from build123d import *

# Parameters (mm, degrees)
BOSS_EXTRUDE1_DEPTH     = 50.8
BOSS_EXTRUDE1_2_DEPTH   = 50.8
BOSS_EXTRUDE2_START     = 50.8
BOSS_EXTRUDE2_DEPTH     = 5.08
F_1_4_CLEARANCE_HOLE1_D = 6.7564
F_1_4_CLEARANCE_HOLE2_D = 6.7564


with BuildPart() as part:
    # Sketch1 → Boss-Extrude1 (new body, symmetric)
    with BuildSketch(Plane.XY):
        with BuildLine():
            ThreePointArc((-13.252570374, 55.853277384), (-42.992049277, 38.038177072), (-57.051702131, 6.35))
            Line((-57.051702131, 6.35), (-70.104, 6.35))
            Line((-70.104, 6.35), (-70.104, 0))
            Line((-70.104, 0), (-51.203999954, 0))
            ThreePointArc((-51.203999954, 0), (-40.6228644, 31.171020183), (-13.252570374, 49.459265965))
            Line((-13.252570374, 49.459265965), (-13.252570374, 55.853277384))
        make_face()
    extrude(amount=BOSS_EXTRUDE1_DEPTH, both=True)



with BuildPart() as body_2:
    # Sketch1 → Boss-Extrude1 2 (new body, symmetric)
    with BuildSketch(Plane.XY):
        with BuildLine():
            Line((13.252570374, 55.853277384), (13.252570374, 49.459265965))
            ThreePointArc((13.252570374, 49.459265965), (37.75154872, 34.59292096), (50.42609614, 8.891481281))
            Line((50.42609614, 8.891481281), (70.104, 8.891481281))
            Line((70.104, 8.891481281), (70.104, 15.241481281))
            Line((70.104, 15.241481281), (55.343621713, 15.241481281))
            ThreePointArc((55.343621713, 15.241481281), (39.858360326, 41.310172211), (13.252570374, 55.853277384))
        make_face()
    extrude(amount=BOSS_EXTRUDE1_2_DEPTH, both=True)


with BuildPart() as part_1:
    add(part.part)

    add(body_2.part)  # Boss-Extrude2 merges body 2
    # Sketch1<4> → Boss-Extrude2 (add)
    with BuildSketch(Plane.XY.offset(BOSS_EXTRUDE2_START)):
        with BuildLine():
            Line((-13.252570374, 55.853277384), (-13.252570374, 49.459265965))
            ThreePointArc((-13.252570374, 49.459265965), (0, 51.203999954), (13.252570374, 49.459265965))
            Line((13.252570374, 49.459265965), (13.252570374, 55.853277384))
            ThreePointArc((13.252570374, 55.853277384), (0, 57.404), (-13.252570374, 55.853277384))
        make_face()
    extrude(amount=-BOSS_EXTRUDE2_DEPTH)

    # 1/4 Clearance Hole1 (through all)
    with Locations(Plane(origin=(0, 6.35, 0), x_dir=(1, 0, 0), z_dir=(0, 1, 0))):
        with Locations((-62.484, -31.75), (-62.484, 31.75)):
            Hole(F_1_4_CLEARANCE_HOLE1_D / 2)

    # 1/4 Clearance Hole2 (through all)
    with Locations(Plane(origin=(0, 15.241481281, 0), x_dir=(1, 0, 0), z_dir=(0, 1, 0))):
        with Locations((62.484, -31.75), (62.484, 31.75)):
            Hole(F_1_4_CLEARANCE_HOLE2_D / 2)


solid = part_1.part
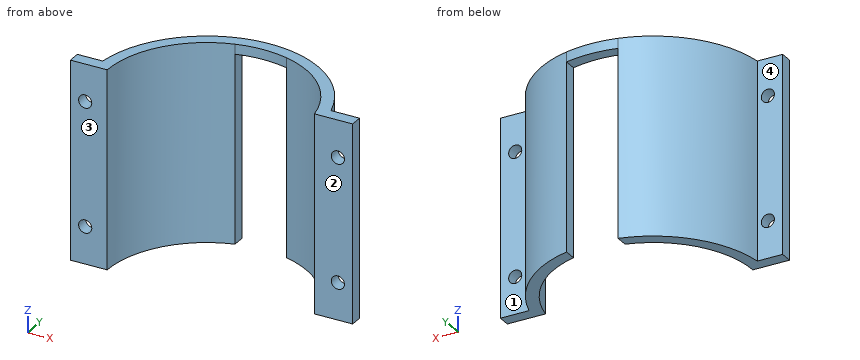
Geometry: final body of the model. Coordinates: model frame, mm. Face numbers are marked on the shaded views. A direction names the side the tool comes from. Give positions to 0.01 mm unless a question says otherwise; leave off trailing zeros. Write each loop counter-clockwise with the first axis right and the second up, starting at its lowest first coordinate (ties: lowest second). Pieces come first, ordered by that corner, then holes.
(1) Cut plane B-B, the plane y = 11. Return loops of the section in (x, z).
(2) Ray query, line 1 (X direction, y = 13, z = -31); line 2 (X direction, y = 13.5, z = -31.75); line 3 (X direction, y = 13, z = 1.5). Return the intervals inside material, ascending.
(3) First-contact query: P1, Ø8, axis at y = 26, z = 39, coming from the -X side; P2, Ø6.5, axis at x = -5.5, y = 52.5, coming from the -Z side; P3, Ø3, axis at y = 46, z = -37, coming from the +X side; P4, Ø10, axis at y = 18, z = 36, coming from the +X side. Flat tips, straight axial feed; report the tip coordinate or a pass-through.
(4) Cut plane A-A, the plane z = -31.75. Return loops of the section in (x, y), then the cut area to 3 significant figures.
(5) Cut plane D-D, the plane z = -0.5. Return loops of the section in (x, y), then the cut area to 3 significant figures.
(6) Cut plane C-C, the plane x = -61. Return loops of the section in (y, z).
(7) Access query for the marked faces 1, 2, 3 and 4. Directions: +Z, -Z, +X, -X, +Y, -Y. A direction counts if a zero-diameter tool reaches every point of the face in a straight line with its end or side. Return the directions, or none.
Values follow:
1. outline: (-56.34, -50.8) - (-50.01, -50.8) - (-50.01, 50.8) - (-56.34, 50.8) - close; (50.01, -50.8) - (70.1, -50.8) - (70.1, 50.8) - (50.01, 50.8) - close; hole circle Ø6.76 at (62.48, -31.75); hole circle Ø6.76 at (62.48, 31.75)
2. line 1: x = -55.91 to -49.53, 49.53 to 59.19, 65.78 to 70.1
2. line 2: x = -55.79 to -49.39, 49.39 to 59.11, 65.86 to 70.1
2. line 3: x = -55.91 to -49.53, 49.53 to 70.1
3. P1: stops at x = -53.02
3. P2: stops at z = 45.72
3. P3: stops at x = 36.26
3. P4: stops at x = 70.1
4. outline: (-70.1, 0) - (-65.86, 0) - (-65.86, 6.35) - (-70.1, 6.35) - close; (-59.11, 0) - (-51.2, 0) arc R51.2 cw to (-13.25, 49.46) - (-13.25, 55.85) arc R57.4 ccw to (-57.05, 6.35) - (-59.11, 6.35) - close; (13.25, 49.46) arc R51.2 cw to (50.43, 8.89) - (59.11, 8.89) - (59.11, 15.24) - (55.34, 15.24) arc R57.4 ccw to (13.25, 55.85) - close; (65.86, 8.89) - (70.1, 8.89) - (70.1, 15.24) - (65.86, 15.24) - close
4. area: 921 mm2
5. outline: (-70.1, 0) - (-51.2, 0) arc R51.2 cw to (-13.25, 49.46) - (-13.25, 55.85) arc R57.4 ccw to (-57.05, 6.35) - (-70.1, 6.35) - close; (13.25, 49.46) arc R51.2 cw to (50.43, 8.89) - (70.1, 8.89) - (70.1, 15.24) - (55.34, 15.24) arc R57.4 ccw to (13.25, 55.85) - close
5. area: 1,010 mm2
6. outline: (0, -50.8) - (6.35, -50.8) - (6.35, -34.78) - (0, -34.78) - close; (0, -28.72) - (6.35, -28.72) - (6.35, 28.72) - (0, 28.72) - close; (0, 34.78) - (6.35, 34.78) - (6.35, 50.8) - (0, 50.8) - close
7. face 1: +Z, -Z, +X, +Y
7. face 2: +Z, -Z, +X, -Y
7. face 3: +Z, -Z, +X, -X, -Y
7. face 4: +Z, -Z, -X, +Y
